```python
from build123d import *

# Parameters (mm, degrees)
SALIENTE_EXTRUIR1_DEPTH    = 15
SALIENTE_EXTRUIR1_2_DEPTH  = 15
SALIENTE_EXTRUIR1_3_DEPTH  = 15
SALIENTE_EXTRUIR1_4_DEPTH  = 15
CORTAR_EXTRUIR1_REACH      = 68.288
CORTAR_EXTRUIR1_END_RADIUS = 40
CROQUIS3_W                 = 25
CROQUIS3_H                 = 10


with BuildPart() as part:
    # Croquis1 → Saliente-Extruir1 (new body)
    with BuildSketch(Plane.XY):
        with BuildLine():
            Line((-4.324392398, 38.256367187), (-4.492875219, 39.746875))
            ThreePointArc((-4.492875219, 39.746875), (-29.830479453, 26.648498937), (-40, 0))
            Line((-40, 0), (-38.5, 0))
            ThreePointArc((-38.5, 0), (-28.711836473, 25.649180227), (-4.324392398, 38.256367187))
        make_face()
    extrude(amount=SALIENTE_EXTRUIR1_DEPTH)



with BuildPart() as body_2:
    # Croquis1 → Saliente-Extruir1 2 (new body)
    with BuildSketch(Plane.XY):
        with BuildLine():
            Line((-38.256367187, -4.324392398), (-39.746875, -4.492875219))
            ThreePointArc((-39.746875, -4.492875219), (-26.648498937, -29.830479453), (0, -40))
            Line((0, -40), (0, -38.5))
            ThreePointArc((0, -38.5), (-25.649180227, -28.711836473), (-38.256367187, -4.324392398))
        make_face()
    extrude(amount=SALIENTE_EXTRUIR1_2_DEPTH)


with BuildPart() as body_3:
    # Croquis1 → Saliente-Extruir1 3 (new body)
    with BuildSketch(Plane.XY):
        with BuildLine():
            ThreePointArc((39.746875, 4.492875219), (26.648498937, 29.830479453), (0, 40))
            Line((0, 40), (0, 38.5))
            ThreePointArc((0, 38.5), (25.649180227, 28.711836473), (38.256367187, 4.324392398))
            Line((38.256367188, 4.324392398), (39.746875, 4.492875219))
        make_face()
    extrude(amount=SALIENTE_EXTRUIR1_3_DEPTH)


with BuildPart() as body_4:
    # Croquis1 → Saliente-Extruir1 4 (new body)
    with BuildSketch(Plane.XY):
        with BuildLine():
            ThreePointArc((4.492875219, -39.746875), (29.830479453, -26.648498937), (40, 0))
            Line((40, 0), (38.5, 0))
            ThreePointArc((38.5, 0), (28.711836473, -25.649180227), (4.324392398, -38.256367188))
            Line((4.324392398, -38.256367188), (4.492875219, -39.746875))
        make_face()
    extrude(amount=SALIENTE_EXTRUIR1_4_DEPTH)


with BuildPart() as part_1:
    add(part.part)

    add(body_2.part)  # Revoluci_n1 merges body 2

    add(body_3.part)  # Revoluci_n1 merges body 3

    add(body_4.part)  # Revoluci_n1 merges body 4
    # Croquis2 → Revoluci_n1 (revolve)
    with BuildSketch(Plane(origin=(0, 0, 0), x_dir=(1, 0, 0), z_dir=(0, 1, 0)), mode=Mode.PRIVATE) as revoluci_n1_sk:
        Polygon((-40, 0), (-45.656854249, 5.656854249), (-43.535533906, 7.778174593), (-35.757359313, 0), align=None)
    revolve(revoluci_n1_sk.sketch.rotate(Axis((0, 0, 0), (0, 0, -1)), 180), axis=Axis((0, 0, 0), (0, 0, -1)))

    # Cortar-Extruir1: up to this cylinder (the profile starts inside it)
    cortar_extruir1_end = Plane(origin=(0, 0, 8), z_dir=(0, 0, -1)) * Cylinder(CORTAR_EXTRUIR1_END_RADIUS, 217.576, mode=Mode.PRIVATE)
    # Croquis3 → Cortar-Extruir1 (cut, up to the surface)
    with BuildSketch(Plane(origin=(0, 0, 0), x_dir=(1, 0, 0), z_dir=(0, 1, 0)), mode=Mode.PRIVATE) as cortar_extruir1_sk1:
        with Locations((-17.5, -8)):
            Rectangle(CROQUIS3_W, CROQUIS3_H)
    cortar_extruir1_tool1 = extrude(cortar_extruir1_sk1.sketch, amount=-CORTAR_EXTRUIR1_REACH, mode=Mode.PRIVATE) & cortar_extruir1_end
    add(cortar_extruir1_tool1.solids().sort_by_distance((-17.5, 0, 8))[0], mode=Mode.SUBTRACT)


solid = part_1.part
```
CAD build for the part. Positions are in the model's coordinates, mm. A direction names the side the tool comes from. Round coordinates to 2 decimals unless told otherwise and drop trailing zeros. Order: outer loops, then holes, each group sorted by start corner. A loop starts at its lowest first (then second) coordinate and runs counter-clockwise, first axis right, second up. Notation, with made-up numbers: (-21, -13.5) - (30, -13.5) arc R31 cw to (30, 11.5) - close; hole circle Ø11 at (-40, 76). An arc over 180 degrees is marked (long way). Answer in a Markdown table with one row per item. Add a question column.
(1) 3-axis set-ups, long thin cutter, end or side, ignore diameter. For faces 4 (the face through (25.355, 28.972, 7.395)), 5 (the face through (-30, -25, 8)), 6 (the face through (29.56, -26.95, 7.4)), 7 (the face through (-31.37, -24.82, 7.4)): which of +Z, -Z, +X, -X, +Y, -Y reach the whole face in a straight line?
(2) Band-saw the part on B-B on y = -32. Count the separate pieces of the cut face and the enclosed holes in it, and give its area (3 significant figures).
(3) Mould opens along Y. For faces 1 (the face through (-18.5, -34.2, 3)), 2 (the face through (38.49, -12.121, -0.354)), 3 (the face through (-29.7, -24.5, 2.4)) say: +Y half, -Y half, draft (parallel to the pull), parting line (faces both ways), or undercut.
(4) Probe L1, parallel to Y at x = 36.5, z = -5.5; L2, parallel to Y at x = 32.5, z = 1; L3, parallel to X at y = 9, z = 9. List the from-to ranges inside material, lowest first. Write a range as [from, to].
(5) Band-saw the part on A-A on z = 9. List the corners of the cut face in (x, y).
(6) Drop flat-ended pins along their axis: pin 1 Ø3 at (x, z) = (6.5, -1) entering from +Y; pin 2 Ø12 at (x, y) = (34.5, -5.5) entering from -Z; pin 3 Ø4 at (x, y) = (-28, 28) entering from -Z; pin 4 Ø12.5 at (x, y) = (-13.5, -33.5) entering from +Z. Give the stop position or say it passes through.
Data:
| question | item | result |
|---|---|---|
| 1 | face 4 | +Z |
| 1 | face 5 | -Y |
| 1 | face 6 | +Z, +X, -Y |
| 1 | face 7 | +Z, -X, -Y |
| 2 | separate pieces | 3 |
| 2 | enclosed holes | 0 |
| 2 | area | 144 mm^2 |
| 3 | face 1 | draft |
| 3 | face 2 | parting line |
| 3 | face 3 | undercut |
| 4 | L1 | y = [-27.17, -19.23], [19.23, 27.17] |
| 4 | L2 | y = [-23.32, -20.64], [20.64, 23.32] |
| 4 | L3 | x = [-38.97, -37.43], [37.43, 38.97] |
| 5 | outline | (-40, 0) - (-38.5, 0) arc R38.5 cw to (-4.32, 38.26) - (-4.49, 39.75) arc R40 ccw to start; (-39.75, -4.49) arc R40 ccw to (-30, -26.46) - (-30, -24.13) arc R38.5 cw to (-38.26, -4.32) - close; (-5, -39.69) arc R40 ccw to (0, -40) - (0, -38.5) arc R38.5 cw to (-5, -38.17) - close; (0, 38.5) arc R38.5 cw to (38.26, 4.32) - (39.75, 4.49) arc R40 ccw to (0, 40) - close; (4.32, -38.26) - (4.49, -39.75) arc R40 ccw to (40, 0) - (38.5, 0) arc R38.5 cw to start |
| 6 | pin 1 | stops at y = 42.02 |
| 6 | pin 2 | stops at z = -5.18 |
| 6 | pin 3 | stops at z = -5.84 |
| 6 | pin 4 | stops at z = 15 |
